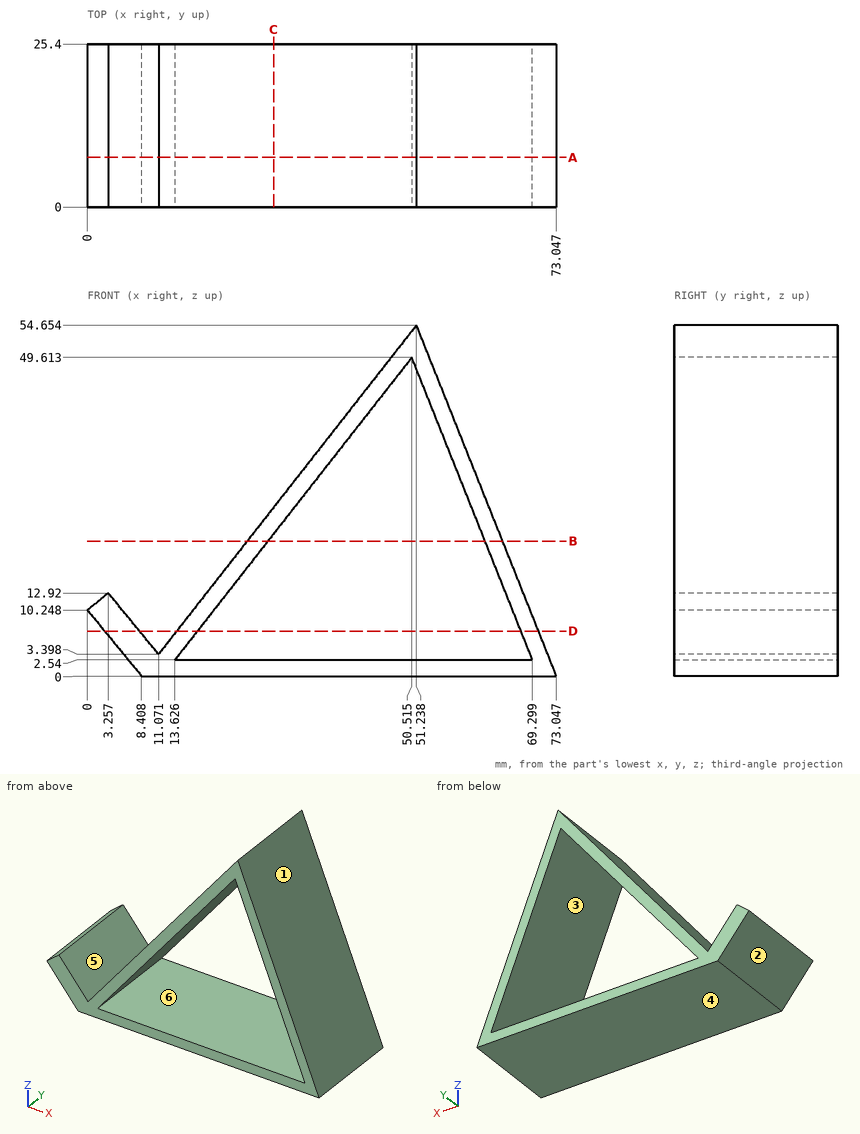
Study the drawing (mm; zero at the part's minimum x, y, z) and answer. A direction names the side the tool comes from. Give positions to 0.01 mm unless a question says otherwise; leave off trailing zeros. Loops run counter-clockwise (first coordinate to the right, second up) from the corner with the lowest first, then second, coordinate; pieces in that order, holes last. Notation, with made-up numbers: (39, -36.75) - (78, -36.75) arc R7 cw to (78, -26.75) - close; hole circle Ø10 at (68.5, 7). An arc over 180 degrees is marked (long way). Answer in a Markdown table with one row per item. Add a question column.
Q1. The part is cut by section C-C (x = 29). Determine the outline of the cut face in (y, z).
Q2. A tool of negligible diameter and unlimited length cuts with its end or side. For the marked faces 5 and 6, from which of +Z, -Z, +X, -X, +Y, -Y can it reach the whole face along a straight path? Write none if from no direction.
Q3. Consider line 1 along X through (y, z) = (15.25, 8) (1 decimal); line 2 along Z through (x, y) = (48, 5.75) (1 decimal); line 3 along X through (y, z) = (11.75, 47) (1 decimal). Determine where each line is inside the solid, lowest interval first.
Q4. The part is cut by section B-B (z = 21). Determine the outline of the cut face in (x, y) (1 decimal).
Q5. The part is cut by section A-A (y = 7.75). Determine the outline of the cut face in (x, z) (1 decimal), and give its area (3 significant figures).
Q6. Determine the mould class of the marked faces 1, 2, 3 and 4 for opening direction X: released by +X, released by -X, zero draft, split by the parting line, or undercut.
Q7. The part is cut by section D-D (z = 7). Determine the outline of the cut face in (x, y) (1 decimal).
Q8. Each of these flat-tipped pins is pushed along its axis until it touches: P1, Ø2, axis at x = 34, y = 10, coming from the +Z side (1 decimal); P2, Ø1.5, axis at x = 19, y = 11, coming from the +Z side (1 decimal); P3, Ø1, axis at y = 22.5, z = 21, coming from the -X side. Where does it stop, or does it pass through?
Solution:
| question | item | result |
|---|---|---|
| 1 | outline | (0, 0) - (25.4, 0) - (25.4, 2.54) - (0, 2.54) - close; (0, 22.16) - (25.4, 22.16) - (25.4, 26.28) - (0, 26.28) - close |
| 2 | face 5 | +Z, +Y, -Y |
| 2 | face 6 | +Y, -Y |
| 3 | line 1 | x = 1.8 to 7.3, 14.7 to 17.9, 67.1 to 69.9 |
| 3 | line 2 | z = 0 to 2.5, 46.4 to 50.5 |
| 3 | line 3 | x = 45.2 to 48.5, 51.6 to 54.3 |
| 4 | outline | (24.9, 0) - (28.1, 0) - (28.1, 25.4) - (24.9, 25.4) - close; (61.9, 0) - (64.7, 0) - (64.7, 25.4) - (61.9, 25.4) - close |
| 5 | outline | (0, 10.2) - (8.4, 0) - (73, 0) - (51.2, 54.7) - (11.1, 3.4) - (3.3, 12.9) - close; hole (13.6, 2.5) - (69.3, 2.5) - (50.5, 49.6) - close |
| 5 | area | 510 mm² |
| 6 | face 1 | released by +X |
| 6 | face 2 | released by -X |
| 6 | face 3 | undercut |
| 6 | face 4 | zero draft |
| 7 | outline | (2.7, 0) - (8.1, 0) - (8.1, 25.4) - (2.7, 25.4) - close; (13.9, 0) - (17.1, 0) - (17.1, 25.4) - (13.9, 25.4) - close; (67.5, 0) - (70.3, 0) - (70.3, 25.4) - (67.5, 25.4) - close |
| 8 | P1 | stops at z = 33.9 |
| 8 | P2 | stops at z = 14.5 |
| 8 | P3 | stops at x = 24.47 |
